```python
from build123d import *

# Parameters (mm, degrees)
SKETCH_R      = 3
PAD_DEPTH     = 4
SKETCH001_R   = 29.5
SKETCH001_R_2 = 3
PAD001_DEPTH  = 25
SKETCH002_R   = 11.5
SKETCH002_R_2 = 3
POCKET_DEPTH  = 18
FILLET_R      = 9
FILLET001_R   = 9


with BuildPart() as part:
    # Sketch → Pad (new body)
    with BuildSketch(Plane.XY):
        Polygon((75, -90), (45, -90), (15, -40), (-15, -40), (-45, -90), (-75, -90), (-50, 40), (50, 40), align=None)
        Circle(SKETCH_R, mode=Mode.SUBTRACT)
    extrude(amount=PAD_DEPTH)

    # Sketch001 → Pad001 (join)
    with BuildSketch(Plane.XY):
        Circle(SKETCH001_R)
        Circle(SKETCH001_R_2, mode=Mode.SUBTRACT)
    extrude(amount=PAD001_DEPTH)

    # Sketch002 → Pocket (cut)
    with BuildSketch(Plane.XY):
        Circle(SKETCH002_R)
        Circle(SKETCH002_R_2, mode=Mode.SUBTRACT)
    extrude(amount=POCKET_DEPTH, mode=Mode.SUBTRACT)

    # Fillet
    fillet_edges = [part.edges().sort_by_distance(p)[0] for p in [
        (-29.5, 0, 4),
    ]]
    fillet(fillet_edges, radius=FILLET_R)

    # Fillet001
    fillet001_edges = [part.edges().sort_by_distance(p)[0] for p in [
        (-75, -90, 2),
        (-45, -90, 2),
        (-15, -40, 2),
        (15, -40, 2),
        (45, -90, 2),
        (75, -90, 2),
        (50, 40, 2),
        (-50, 40, 2),
    ]]
    fillet(fillet001_edges, radius=FILLET001_R)


solid = part.part
```
The model under review builds one solid part; all positions refer to its coordinate system, in mm. A direction names the side the tool comes from. Give positions to 0.01 mm unless a question says otherwise; leave off trailing zeros. Write each loop counter-clockwise with the first axis right and the second up, starting at its lowest first coordinate (ties: lowest second). Pieces come first, ordered by that corner, then holes. Notation, with made-up numbers: M 7,88.25 L 28,88.25 A15 cw 28,117.25 Z; hole C -24.5,23.5 d2. An arc over 180 degrees is marked long. Write each question's results on one line, items separated by ' | '. Start each with the question number.
1. Insertion check: pin 1 Ø3 at (x, z) = (0, 1.5) entering from -Y; pin 2 Ø4 at (y, z) = (-51, 5.5) entering from +X; pin 3 Ø12 at (x, z) = (18.5, 9) entering from +Y; pin 4 Ø1.5 at (x, z) = (26, 17.5) entering from -Y. Each pin has a flat end and moves straight along its axis. Give the tip position at first contact, or say it passes through.
2. We need section B-B (y = -64). Write out the cut boundary in (x, z).
3. We need section D-D (y = 0). Write out the cut boundary in (x, z).
4. Mouldability with a two-part tool opening along Y and no side actions: class faces 4 (the flat face through (2.4, -2.4, 18)), 5 (the cylindrical face through (48.364, 37.883, 2.028)), 6 (the flat face through (57, -90, 2)) as released by +Y, released by -Y, zero draft, split by the parting line, or undercut.
5. We need section A-A (x = 0). Write out the cut boundary in (y, z), and give its area (3 significant figures).
6. We need section C-C (x = -61). Write out the cut boundary in (y, z).
7. For probe 1 along Y at (x, z) = (0, 23.5); probe 2 along Z at (x, y) = (-54.5, -29); probe 3 along Y at (x, z) = (0, 3.5), list the stretches that pass through material, from the lowest coordinate up. Write a range as [from, to].
8. For faces 1 (the cylindrical face through (45.718, -88.864, 2.028)), 2 (the cylindrical face through (28.14, 8.86, 18.92)), 3 (the cylindrical face through (-1.5, 11.4, 8.9)), list the 3-axis set-ups (+Z, -Z, +X, -X, +Y, -Y) from which the entire face can be reached by the end or side of a thin tool; tool diameter is ignored.
Results found:
1) pin 1: stops at y = -40 | pin 2: stops at x = 67.75 | pin 3: stops at y = 40 | pin 4: stops at y = -15.25
2) outline: M -70,0 L -29.4,0 L -29.4,4 L -70,4 Z; M 29.4,0 L 70,0 L 70,4 L 29.4,4 Z
3) outline: M -57.69,0 L -11.5,0 L -11.5,18 L -3,18 L -3,25 L -29.5,25 L -29.5,13 A9 cw -38.5,4 L -57.69,4 Z; M 3,18 L 11.5,18 L 11.5,0 L 57.69,0 L 57.69,4 L 38.5,4 A9 cw 29.5,13 L 29.5,25 L 3,25 Z
4) face 4: undercut | face 5: released by +Y | face 6: released by -Y
5) outline: M -40,0 L -11.5,0 L -11.5,18 L -3,18 L -3,25 L -29.5,25 L -29.5,13 A9 cw -38.5,4 L -40,4 Z; M 3,18 L 11.5,18 L 11.5,0 L 40,0 L 40,4 L 38.5,4 A9 cw 29.5,13 L 29.5,25 L 3,25 Z | area: 1,140 mm^2
6) outline: M -90,0 L -17.2,0 L -17.2,4 L -90,4 Z
7) probe 1: y = [-29.5, -3], [3, 29.5] | probe 2: z = [0, 4] | probe 3: y = [-40, -11.5], [11.5, 40]
8) face 1: +Z, -Z, -Y | face 2: +Z | face 3: -Z
